Autodesk Inventor part; units mm, degrees
ref_plane "工作平面2" through (0, -8, 0) normal (0, -1, 0) x (1, 0, 0)
ref_plane "工作平面1" through (0, -10, 0) normal (0, -1, 0) x (1, 0, 0)
ref_plane "工作平面3" through (0, -16, 0) normal (0, -1, 0) x (1, 0, 0)
sketch "草图1" plane through (0, 0, 0) normal (0, 1, 0) x (-1, 0, 0)
  circle A0 centre (0, 0) radius 12.5
  circle A1 centre (0, 0) radius 5.8
  dimension "d0" = 25
  dimension "d1" = 11.6
extrude "拉伸1" add sketch "草图1" along normal blind 3.5 contours A0 | A1
extrude "拉伸2" add sketch "草图1" against normal blind 6 contours A1
ref_plane "工作平面2" through (0, -8, 0) normal (0, -1, 0) x (1, 0, 0)
sketch "草图3" plane through (0, -8, 0) normal (0, -1, 0) x (1, 0, 0)
  circle A0 centre (0, 0) radius 5
  dimension "d10" = 10
ref_plane "工作平面1" through (0, -10, 0) normal (0, -1, 0) x (1, 0, 0)
sketch "草图2" plane through (0, -10, 0) normal (0, -1, 0) x (1, 0, 0)
  circle A0 centre (0, 0) radius 5.8
extrude "拉伸3" add sketch "草图2" along normal blind 6
loft "放样1" add profiles "草图3" section 1 edges at (5.8, -6, 0) section 3 edges at (-5.8, -10, 0)
ref_plane "工作平面3" through (0, -16, 0) normal (0, -1, 0) x (1, 0, 0)
sketch "草图4" plane through (0, -16, 0) normal (0, -1, 0) x (1, 0, 0)
  circle A0 centre (0, 0) radius 3.8
  dimension "d18" = 7.6
extrude "拉伸4" add sketch "草图4" along normal blind 12
chamfer "倒角1" distance 1 angle 45 1 edges at (-3.8, -28, 0)
chamfer "倒角2" distance 2 angle 45 1 edges at (12.5, 3.5, 0)
sketch "草图5" plane through (0, 3.5, 0) normal (0, 1, 0) x (1, 0, 0)
  circle A0 centre (0, 0) radius 3.1
  line L0 (-3.0786, -1.8264) -> (-3.121, 1.7529)
  line L1 (-3.121, 1.7529) -> (-0.0425, 3.5793)
  line L2 (-0.0425, 3.5793) -> (3.0786, 1.8264)
  line L3 (3.0786, 1.8264) -> (3.121, -1.7529)
  line L4 (3.121, -1.7529) -> (0.0425, -3.5793)
  line L5 (0.0425, -3.5793) -> (-3.0786, -1.8264)
  dimension "d29" = 6.2
extrude "拉伸5" cut sketch "草图5" against normal blind 5
chamfer "倒角3" distance 0.5 angle 45 6 edges at (3.0998, 3.5, -0.0368) (1.5181, 3.5, -2.7029) (-1.5817, 3.5, -2.6661) (-3.0998, 3.5, 0.0368) (-1.5181, 3.5, 2.7029) (1.5817, 3.5, 2.6661)
thread "螺纹2"
properties part number "Spindle_Screw"
Design review of the part built by this model. Coordinates are the model's own, in mm. A direction names the side the tool comes from. Coordinates: 2 decimals unless noted, no trailing zeros. Loops run counter-clockwise (first coordinate to the right, second up) from the corner with the lowest first, then second, coordinate; pieces in that order, holes last.
Item 1: Draft analysis for pull direction X (two halves, no side actions). For faces 4 (the flat face through (-1.664, 3.246, 2.904)), 5 (the cylindrical face through (-3.796, -21.423, -0.167)), 6 (the flat face through (-2.6, 0, -5.4)), state which applies: pulls with the +X half, pulls with the -X half, needs draft (parallel to the pull), parting line crosses it, or undercut.
Completed:
face 4: undercut
face 5: parting line crosses it
face 6: needs draft
Item 2: Add section B-B (y = -12). Write out the cut boundary in (x, z), and give its area (3 significant figures).
Completed:
outline: circle Ø11.6 at (0, 0)
area: 106 mm2
Item 3: Wall thickness on L1, parallel to Y at x = 1.75, z = -7.75; L2, parallel to Z at x = -0.25, y = -24; L3, parallel to Z at x = 0.75, y = 1.5: over which ranges is each line inside the solid? List them lowest first.
Completed:
L1: y = 0 to 3.5
L2: z = -3.79 to 3.79
L3: z = -12.48 to -3.13, 3.16 to 12.48
Item 4: For faces 1 (the flat face through (1.664, 3.246, -2.904)), 2 (the cylindrical face through (5.794, -2.958, 0.255)), 3 (the flat face through (0, -28, 0)), list the 3-axis set-ups (+Z, -Z, +X, -X, +Y, -Y) from which the entire face can be reached by the end or side of a thin tool; tool diameter is ignored.
Completed:
face 1: +Y
face 2: -Y
face 3: +Z, -Z, +X, -X, -Y
Item 5: Add section A-A (y = -23). Write out the cut boundary in (x, z), and give its area (3 significant figures).
Completed:
outline: circle Ø7.6 at (0, 0)
area: 45.4 mm2
Item 6: Clearance check with flat-ended pins moving along their axes: pin 1 (3 mm diameter, centred on y = -23, z = 0.5, fed in from +X); pin 2 (2 mm diameter, centred on x = -7.5, y = -12.5, fed in from +Z); pin 3 (8 mm diameter, centred on x = -2.5, y = -17.5, fed in from -Z); pin 4 (12.5 mm diameter, centred on x = -2.5, z = -2.5, fed in from -Y). State where each tip first meets the part, or that it passes through.
Completed:
pin 1: stops at x = 3.8
pin 2: passes through
pin 3: stops at z = -5.8
pin 4: stops at y = -28
